```python
from build123d import *

# Parameters (mm, degrees)
SKETCH_1_R          = 1.462780711
SKETCH_1_R_2        = 1.582906388
SKETCH_1_R_3        = 1.5
SKETCH_1_R_4        = 1.65
EXTRUDE_1_DEPTH     = 4
SKETCH_3_R          = 3.5
SKETCH_3_R_2        = 1.6
CUT_EXTRUDE_1_DEPTH = 4
SKETCH_4_R          = 4.5
SKETCH_4_R_2        = 2.1
CUT_EXTRUDE_2_DEPTH = 4
CUT_EXTRUDE_7_DEPTH = 4
SKETCH_12_W         = 118
SKETCH_12_H         = 10
CUT_EXTRUDE_8_DEPTH = 4
SKETCH_13_W         = 20
SKETCH_13_H         = 15
SKETCH_13_R         = 1.6
EXTRUDE_4_DEPTH     = 4
FILLET_4_R          = 3
SKETCH_14_W         = 20
SKETCH_14_H         = 30
CUT_EXTRUDE_9_DEPTH = 182.063524764
FILLET_5_R          = 3


with BuildPart() as part:
    # 草图1 → 凸台-拉伸1 (new body)
    with BuildSketch(Plane.XY):
        Polygon((-128, 10), (-128, -10), (-10, -128), (10, -128), (10, 10), align=None)
        with Locations((-44.314491387, -77.548510103)):
            Circle(SKETCH_1_R, mode=Mode.SUBTRACT)
        with Locations((-38.657637138, -71.891655854)):
            Circle(SKETCH_1_R_2, mode=Mode.SUBTRACT)
        with Locations((-77.548510103, -44.314491387)):
            Circle(SKETCH_1_R_3, mode=Mode.SUBTRACT)
        with Locations((-71.891655854, -38.657637138)):
            Circle(SKETCH_1_R_3, mode=Mode.SUBTRACT)
        with Locations((-29.196699141, -46.874368671)):
            Circle(SKETCH_1_R_4, mode=Mode.SUBTRACT)
        with Locations((-46.874368671, -29.196699141)):
            Circle(SKETCH_1_R_4, mode=Mode.SUBTRACT)
        with Locations((-22.125631329, -39.803300859)):
            Circle(SKETCH_1_R_4, mode=Mode.SUBTRACT)
        with Locations((-39.803300859, -22.125631329)):
            Circle(SKETCH_1_R_4, mode=Mode.SUBTRACT)
    extrude(amount=EXTRUDE_1_DEPTH)

    # 草图3 → 切除-拉伸1 (cut)
    with BuildSketch(Plane.XY.offset(4)):
        Circle(SKETCH_3_R)
        with Locations((5, 5)):
            Circle(SKETCH_3_R_2)
        with Locations((-5, 5)):
            Circle(SKETCH_3_R_2)
        with Locations((-5, -5)):
            Circle(SKETCH_3_R_2)
        with Locations((5, -5)):
            Circle(SKETCH_3_R_2)
        with Locations((-20, -5)):
            Circle(SKETCH_3_R_2)
        with Locations((-5, -20)):
            Circle(SKETCH_3_R_2)
        with Locations((5, -20)):
            Circle(SKETCH_3_R_2)
        with Locations((5, 20)):
            Circle(SKETCH_3_R_2)
        with Locations((-5, 20)):
            Circle(SKETCH_3_R_2)
        with Locations((20, -5)):
            Circle(SKETCH_3_R_2)
        with Locations((20, 5)):
            Circle(SKETCH_3_R_2)
        with Locations((-20, 5)):
            Circle(SKETCH_3_R_2)
    extrude(amount=-CUT_EXTRUDE_1_DEPTH, mode=Mode.SUBTRACT)

    # 草图4 → 切除-拉伸2 (cut)
    with BuildSketch(Plane.XY.offset(4)):
        with Locations((0, -60)):
            Circle(SKETCH_4_R)
        with Locations((-5, -29.263884189)):
            Circle(SKETCH_4_R_2)
        with Locations((5, -29.263884189)):
            Circle(SKETCH_4_R_2)
        with Locations((5, -49.263884189)):
            Circle(SKETCH_4_R_2)
        with Locations((5, -69.263884189)):
            Circle(SKETCH_4_R_2)
        with Locations((5, -89.263884189)):
            Circle(SKETCH_4_R_2)
        with Locations((-5, -49.263884189)):
            Circle(SKETCH_4_R_2)
        with Locations((-5, -69.263884189)):
            Circle(SKETCH_4_R_2)
        with Locations((-5, -89.263884189)):
            Circle(SKETCH_4_R_2)
        with Locations(Location((-89.263884189, -5, 0), (0, 0, 180))):
            Circle(SKETCH_4_R_2)
        with Locations(Location((-69.263884189, -5, 0), (0, 0, 180))):
            Circle(SKETCH_4_R_2)
        with Locations(Location((-49.263884189, -5, 0), (0, 0, 180))):
            Circle(SKETCH_4_R_2)
        with Locations(Location((-89.263884189, 5, 0), (0, 0, 180))):
            Circle(SKETCH_4_R_2)
        with Locations(Location((-69.263884189, 5, 0), (0, 0, 180))):
            Circle(SKETCH_4_R_2)
        with Locations(Location((-49.263884189, 5, 0), (0, 0, 180))):
            Circle(SKETCH_4_R_2)
        with Locations(Location((-29.263884189, 5, 0), (0, 0, 180))):
            Circle(SKETCH_4_R_2)
        with Locations(Location((-29.263884189, -5, 0), (0, 0, 180))):
            Circle(SKETCH_4_R_2)
        with Locations(Location((-60, 0, 0), (0, 0, 180))):
            Circle(SKETCH_4_R)
    extrude(amount=-CUT_EXTRUDE_2_DEPTH, mode=Mode.SUBTRACT)

    # 草图11 → 切除-拉伸7 (cut)
    with BuildSketch(Plane.XY.offset(4)):
        Polygon((-69, -69), (-64.050252532, -64.050252532), (-99.405591591, -28.694913472), (-104.355339059, -33.644660941), align=None)
        Polygon((-28.694913472, -99.405591591), (-64.050252532, -64.050252532), (-69, -69), (-33.644660941, -104.355339059), align=None)
    extrude(amount=-CUT_EXTRUDE_7_DEPTH, mode=Mode.SUBTRACT)

    # 草图12 → 切除-拉伸8 (cut)
    with BuildSketch(Plane.XY.offset(4)):
        with Locations((-69, 5)):
            Rectangle(SKETCH_12_W, SKETCH_12_H)
    extrude(amount=-CUT_EXTRUDE_8_DEPTH, mode=Mode.SUBTRACT)

    # 草图13 → 凸台-拉伸4 (add)
    with BuildSketch(Plane.XY.offset(4)):
        with Locations((0, 17.5)):
            Rectangle(SKETCH_13_W, SKETCH_13_H)
        with Locations((-5, 20)):
            Circle(SKETCH_13_R, mode=Mode.SUBTRACT)
        with Locations((5, 20)):
            Circle(SKETCH_13_R, mode=Mode.SUBTRACT)
    extrude(amount=-EXTRUDE_4_DEPTH)

    # 圆角4
    fillet_4_edges = [part.edges().sort_by_distance(p)[0] for p in [
        (-99.405591591, -28.694913472, 2),
        (-28.694913472, -99.405591591, 2),
        (-33.644660941, -104.355339059, 2),
        (-104.355339059, -33.644660941, 2),
        (-64.5, 0, 2),
        (-55.5, 0, 2),
        (-10, 0, 2),
        (-128, 0, 2),
        (10, -128, 2),
        (-10, -128, 2),
        (-128, -10, 2),
        (10, 25, 2),
        (-10, 25, 2),
    ]]
    fillet(fillet_4_edges, radius=FILLET_4_R)

    # 草图14 → 切除-拉伸9 (cut, through all)
    with BuildSketch(Plane(origin=(0, 0, 0), x_dir=(-1, 0, 0), z_dir=(0, 0, -1))):
        with Locations((0, 25)):
            Rectangle(SKETCH_14_W, SKETCH_14_H)
    extrude(amount=-CUT_EXTRUDE_9_DEPTH, mode=Mode.SUBTRACT)

    # 圆角5
    fillet_5_edges = [part.edges().sort_by_distance(p)[0] for p in [
        (-10, 10, 2),
        (10, 10, 2),
    ]]
    fillet(fillet_5_edges, radius=FILLET_5_R)


solid = part.part
```
Part model, mm, in its own coordinate system. Round coordinates to 2 decimals unless told otherwise and drop trailing zeros. Loops run counter-clockwise (first coordinate to the right, second up) from the corner with the lowest first, then second, coordinate; pieces in that order, holes last.
1. Drill centre lines: line 1 along X through (y, z) = (-28, 2.6); line 2 along X through (y, z) = (-39, 2.3); line 3 along X through (y, z) = (-89, 1.75). Where is each one in solid material? Low to high.
Solutions:
line 1: x = -110 to -48.01, -45.74 to -6.68, -3.32 to 3.32, 6.68 to 10
line 2: x = -89.1 to -73.35, -70.43 to -23.57, -20.68 to 10
line 3: x = -39.1 to -7.08, -2.92 to 2.92, 7.08 to 10
2. Slice it at A-A (x = 0). Give the cut face in (y, z).
Solutions:
outline: (-128, 0) - (-64.5, 0) - (-64.5, 4) - (-128, 4) - close; (-55.5, 0) - (-3.5, 0) - (-3.5, 4) - (-55.5, 4) - close; (3.5, 0) - (10, 0) - (10, 4) - (3.5, 4) - close
3. Flat gauge pins, fed straight in: pin 1 (2 mm diameter, centred on y = 5.5, z = 1, fed in from -X); pin 2 (2 mm diameter, centred on x = -35, z = 1.5, fed in from +Y). Where does each tip first touch, or does it go through?
Solutions:
pin 1: stops at x = -10
pin 2: stops at y = 0
4. Slice it at C-C (z = 1). Count the separate pieces of the cut face and the enclosed holes in it, and give its area (3 significant figures).
Solutions:
separate pieces: 1
enclosed holes: 29
area: 9,770 mm2
5. Slice it at D-D (x = -81). Give the cut face in (y, z).
Solutions:
outline: (-47.1, 0) - (0, 0) - (0, 4) - (-47.1, 4) - close
6. Two-plate mould, pull along Y, no slides. Class faces 1 (the face through (10, -60, 2)), 2 (the face through (-10.86, 0.9, 1.97)), 3 (the face through (-99.373, -29.938, 1.972)), 4 (the face through (-5.455, -31.314, 2.028)): pulls with the +Y half, pulls with the -Y half, needs draft (parallel to the pull), parting line crosses it, or undercut.
Solutions:
face 1: needs draft
face 2: pulls with the +Y half
face 3: pulls with the -Y half
face 4: undercut
7. Slice it at B-B (x = -16). Give the cut face in (y, z), and give its area (3 significant figures).
Solutions:
outline: (-122, 0) - (0, 0) - (0, 4) - (-122, 4) - close
area: 488 mm2
